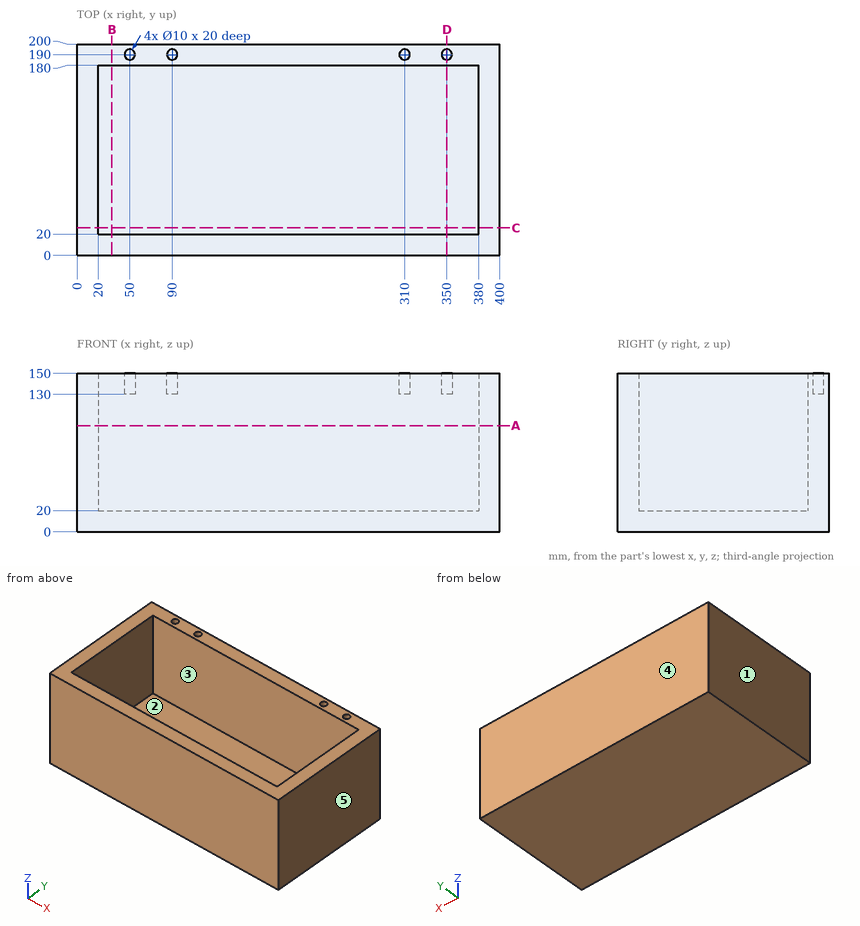
Check sheet for the drawn part. Datum: minimum x, y, z corner. Units: mm. A direction names the side the tool comes from. Give positions to 0.01 mm unless a question says otherwise; leave off trailing zeros. Order: outer loops, then holes, each group sorted by start corner. A loop starts at its lowest first (then second) coordinate and runs counter-clockwise, first axis right, second up. Notation, with made-up numbers: (16, 28.5) -> (53, 28.5) arc R16 cw to (53, 52.5) -> close; hole circle Ø1 at (37.5, 45.25). An arc over 180 degrees is marked (long way). One line per item, written item: value.
(1) Scan lines: line 1 along X through (y, z) = (190, 143.25); line 2 along Y through (x, z) = (90, 135.5); line 3 along Y through (x, z) = (180, 64.5). Record each from-to range of solid material in increasing order. Write a range as [from, to].
Final values:
line 1: [0, 45], [55, 85], [95, 305], [315, 345], [355, 400]
line 2: [0, 20], [180, 185], [195, 200]
line 3: [0, 20], [180, 200]
(2) Gauge pin test, flat ends, axial feed: pin 1 (3 mm diameter, centred on x = 310, y = 190, fed in from +Z); pin 2 (4 mm diameter, centred on x = 245, y = 164, fed in from +Z); pin 3 (13 mm diameter, centred on x = 310, y = 190, fed in from -Z). Record the tip position at first contact, or that the pin passes through.
Final values:
pin 1: z = 130
pin 2: z = 20
pin 3: z = 0
(3) Sectioned sample at D-D on x = 350. Record the cut outline in (y, z), then the cut area to 3 significant figures.
Final values:
outline: (0, 0) -> (200, 0) -> (200, 150) -> (195, 150) -> (195, 130) -> (185, 130) -> (185, 150) -> (180, 150) -> (180, 20) -> (20, 20) -> (20, 150) -> (0, 150) -> close
area: 9,000 mm^2
(4) Sectioned sample at A-A on z = 100.5. Record the cut outline in (x, y), then the cut area to 3 significant figures.
Final values:
outline: (0, 0) -> (400, 0) -> (400, 200) -> (0, 200) -> close; hole (20, 20) -> (380, 20) -> (380, 180) -> (20, 180) -> close
area: 22,400 mm^2
(5) Tool access check on the marked faces 1 and 2. Record the directions out of +Z, -Z, +X, -X, +Y, -Y that give a thin tool (end or side, any length) a straight path to the whole face; none if there is none.
Final values:
face 1: +Z, -Z, -X, +Y, -Y
face 2: +Z
(6) Sectioned sample at C-C on y = 26. Record the cut outline in (x, z).
Final values:
outline: (0, 0) -> (400, 0) -> (400, 150) -> (380, 150) -> (380, 20) -> (20, 20) -> (20, 150) -> (0, 150) -> close
(7) Draft check along Y on the marked faces 3, 4 and 5. Enter one of: pulls with the +Y half, pulls with the -Y half, needs draft (parallel to the pull), parting line crosses it, or undercut.
Final values:
face 3: undercut
face 4: pulls with the +Y half
face 5: needs draft
(8) Sectioned sample at B-B on x = 33. Record the cut outline in (y, z), then the cut area to 3 significant figures.
Final values:
outline: (0, 0) -> (200, 0) -> (200, 150) -> (180, 150) -> (180, 20) -> (20, 20) -> (20, 150) -> (0, 150) -> close
area: 9,200 mm^2
